For this review, use the dimensioned drawing (mm, ordinates from the lowest corner) and the shaded views. A direction names the side the tool comes from. Give positions to 0.01 mm unless a question says otherwise; leave off trailing zeros. Write each loop counter-clockwise with the first axis right and the second up, starting at its lowest first coordinate (ties: lowest second). Pieces come first, ordered by that corner, then holes. Notation, with made-up numbers: (10, 89.5) - (21, 89.5) arc R10 cw to (21, 100.5) - close; hole circle Ø4 at (-39, -34). An arc over 180 degrees is marked (long way). One line per question, with ' | ' between items. Start each with the question number.
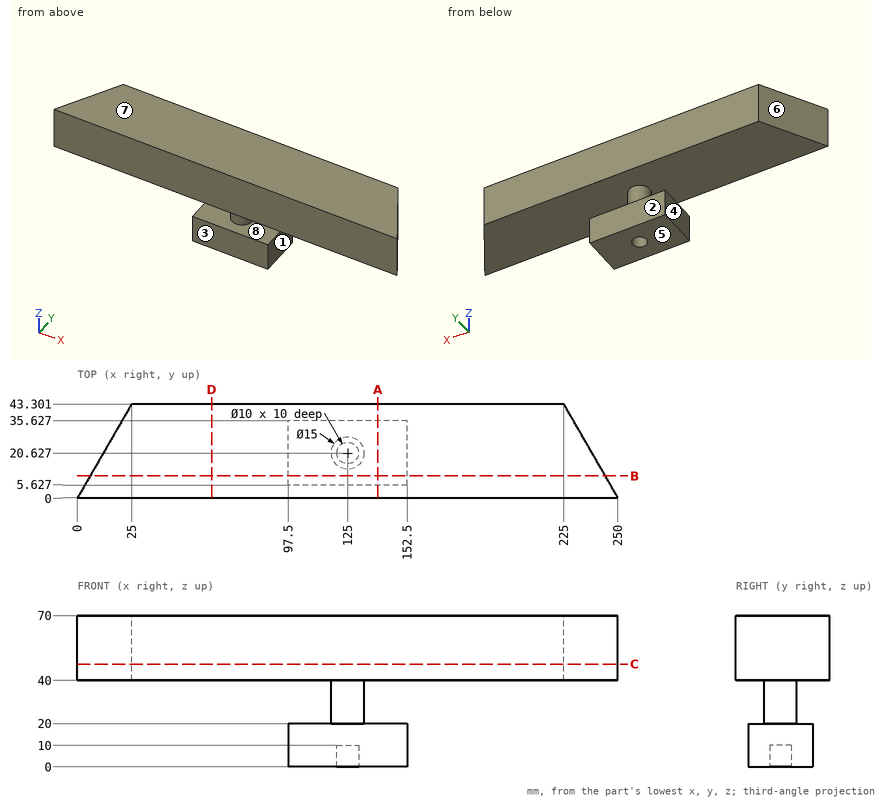
Item 1: Take a section at A-A (x = 139). Give the boundary of the cut face in (y, z).
Item 2: The part is to be moulded in two halves that separate along Z. For the marked faces 5, 6, 7 and 8, say which applies: +Z half, -Z half, draft (parallel to the pull), parting line (faces both ways), or undercut.
Item 3: Clearance check with flat-ended pins moving along their axes: P1, Ø6, axis at y = 13.5, z = 17.5, coming from the -X side; P2, Ø8, axis at x = 125, y = 20.63, coming from the -Z side; P3, Ø5, axis at y = 18.5, z = 28, coming from the +X side; P4, Ø6, axis at x = 178, z = 44.5, coming from the -Y side. State where each tip first meets the part, or that it passes through.
Item 4: Machinability: for the marked faces 1, 2, 3 and 4, which of the approach directions +Z, -Z, +X, -X, +Y, -Y give a long, thin tool a straight path to every point of the face, cutting with its end or side? Answer none if there is none.
Item 5: For probe 1 along Y at (x, z) = (125, 5); probe 2 along Z at (x, y) = (136.5, 31.5); probe 3 along Z at (x, y) = (81, 9), list the stretches that pass through material, from the lowest coordinate up.
Item 6: Take a section at C-C (z = 47.5). Give the boundary of the cut face in (x, y).
Item 7: Take a section at B-B (y = 10). Give the boundary of the cut face in (x, z).
Item 8: Take a section at D-D (x = 62). Give the boundary of the cut face in (y, z).
Check sheet entries:
1) outline: (0, 40) - (43.3, 40) - (43.3, 70) - (0, 70) - close; (5.63, 0) - (35.63, 0) - (35.63, 20) - (5.63, 20) - close
2) face 5: -Z half | face 6: draft | face 7: +Z half | face 8: undercut
3) P1: stops at x = 97.5 | P2: stops at z = 10 | P3: stops at x = 132.5 | P4: stops at y = 0
4) face 1: -Z, +X, +Y, -Y | face 2: -Z, +X, -X, +Y | face 3: -Z, +X, -X, -Y | face 4: -Z, -X, +Y, -Y
5) probe 1: y = 5.63 to 15.63, 25.63 to 35.63 | probe 2: z = 0 to 20, 40 to 70 | probe 3: z = 40 to 70
6) outline: (0, 0) - (250, 0) - (225, 43.3) - (25, 43.3) - close
7) outline: (5.77, 40) - (244.23, 40) - (244.23, 70) - (5.77, 70) - close; (97.5, 0) - (152.5, 0) - (152.5, 20) - (97.5, 20) - close
8) outline: (0, 40) - (43.3, 40) - (43.3, 70) - (0, 70) - close
